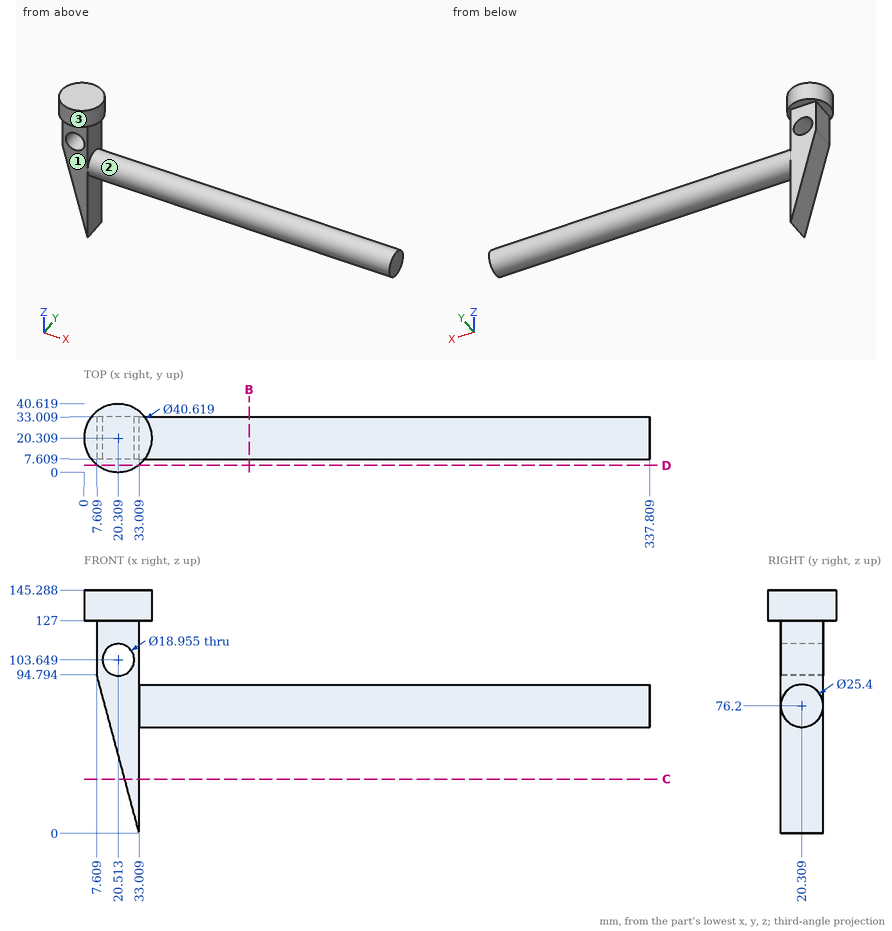
Can you work these out from the drawing? Everything is in mm from the part's minimum corner. A direction names the side the tool comes from. Round coordinates to 2 decimals unless told otherwise and drop trailing zeros. Loops run counter-clockwise (first coordinate to the right, second up) from the corner with the lowest first, then second, coordinate; pieces in that order, holes last. Notation, with made-up numbers: (10, 41.5) - (25, 41.5) arc R18 ccw to (25, 56.5) - close; hole circle Ø4 at (40.25, -21.75). An arc over 180 degrees is marked (long way). Answer in a Markdown table with one row per item. Add a question column.
Q1. I want a section at D-D on y = 4. List the corners of the cut face in (x, z) for me, and give its area (3 significant figures).
Q2. I want a section at B-B on x = 98.5. List the corners of the cut face in (y, z) for me, and give its area (3 significant figures).
Q3. I need wall thicknesses on L1, parallel to Z at x = 40, y = 22.5; L2, parallel to Y at x = 26, z = 80; L3, parallel to X at y = 27.5, z = 48. Which ranges of each line are inside material? Lowest first, please.
Q4. I want a section at C-C on z = 32.5. List the corners of the cut face in (x, y) for me, and give its area (3 significant figures).
Q5. Which directions (+Z, -Z, +X, -X, +Y, -Y) give clear straight access to the entire face, cutting with the end or side of a thin tool? Please do the marked faces 1, 2 and 3.
Q6. For pin 1 Ø10 at (x, y) = (78.5, 28) entering from +Z; pin 2 Ø2 at (x, y) = (165.5, 8) entering from +Z; pin 3 Ø2 at (y, z) = (8.5, 77) entering from -X, each with a flat end and sliding along its axis, tell me the tip position at first contact or that it passes through.
A:
| question | item | result |
|---|---|---|
| 1 | outline | (8.21, 127) - (32.41, 127) - (32.41, 145.29) - (8.21, 145.29) - close |
| 1 | area | 443 mm^2 |
| 2 | outline | circle Ø25.4 at (20.31, 76.2) |
| 2 | area | 507 mm^2 |
| 3 | L1 | 63.69 to 88.71, 127 to 145.29 |
| 3 | L2 | 7.61 to 33.01 |
| 3 | L3 | 20.15 to 33.01 |
| 4 | outline | (24.3, 7.61) - (33.01, 7.61) - (33.01, 33.01) - (24.3, 33.01) - close |
| 4 | area | 221 mm^2 |
| 5 | face 1 | -Z, +X, -X, -Y |
| 5 | face 2 | +X |
| 5 | face 3 | +Z |
| 6 | pin 1 | z = 88.61 |
| 6 | pin 2 | z = 81.98 |
| 6 | pin 3 | x = 12.11 |
